from build123d import *

# Parameters (mm, degrees)
SKETCH1_W               = 181
SKETCH1_H               = 90.5
BOSS_EXTRUDE1_DEPTH     = 2.25
SKETCH2_R               = 3.5687
CUT_EXTRUDE1_DEPTH      = 1
CUT_EXTRUDE1_DEPTH_BACK = 91.5


with BuildPart() as part:
    # Sketch1 → Boss-Extrude1 (new body, symmetric)
    with BuildSketch(Plane(origin=(0, 0, 0), x_dir=(0, 0, -1), z_dir=(1, 0, 0))):
        with Locations((0, -45.25)):
            Rectangle(SKETCH1_W, SKETCH1_H)
    extrude(amount=BOSS_EXTRUDE1_DEPTH, both=True)

    # Sketch2 → Cut-Extrude1 (cut, two sides)
    with BuildSketch(Plane(origin=(88.25, 0, 0), x_dir=(0, 0, -1), z_dir=(1, 0, 0))) as cut_extrude1_sk:
        with Locations((0, -69.85)):
            Circle(SKETCH2_R)
        with Locations((69.85, -69.85)):
            Circle(SKETCH2_R)
    extrude(amount=CUT_EXTRUDE1_DEPTH, mode=Mode.SUBTRACT)
    extrude(cut_extrude1_sk.sketch, amount=-CUT_EXTRUDE1_DEPTH_BACK, mode=Mode.SUBTRACT)


solid = part.part
Design review of the part built by this model. Coordinates are the model's own, in mm. Give positions to 0.01 mm unless a question says otherwise; leave off trailing zeros. Loops run counter-clockwise (first coordinate to the right, second up) from the corner with the lowest first, then second, coordinate; pieces in that order, holes last. Notation, with made-up numbers: (80.5, 83) -> (105.5, 83) arc R8 cw to (105.5, 88) -> close; hole circle Ø5 at (43.25, 83.5). An arc over 180 degrees is marked (long way). One line per question, with ' | ' between items. Start each with the question number.
(1) We need section A-A (y = -69.85). State the section outline as (x, z) points, and give its area (3 significant figures).
(2) We need section B-B (z = 0). State the section outline as (x, y) points, and give its area (3 significant figures).
(3) For line 1 (Y direction, x = 0.2, z = -69.85); line 2 (Z direction, x = 0.6, y = -68), list the stretches that pass through material, from the lowest coordinate up.
(4) Insertion check: P1, Ø8, axis at y = -69.85, z = -69.85, coming from the -X side. The pin has a flat end and moves straight along its axis. Give the tip position at first contact, or say it passes through.
(5) Draft analysis for pull direction Y (two halves, no side actions). For faces 1 (the face through (0, -90.5, 1)), 2 (the face through (0.031, -73.016, -71.497)), 3 (the face through (0.031, -73.016, -1.647)), 4 (the face through (0, -46, -90.5)), state which applies: +Y half, -Y half, draft (parallel to the pull), parting line (faces both ways), or undercut.
The answers:
1) outline: (-2.25, -90.5) -> (2.25, -90.5) -> (2.25, -73.42) -> (-2.25, -73.42) -> close; (-2.25, -66.28) -> (2.25, -66.28) -> (2.25, -3.57) -> (-2.25, -3.57) -> close; (-2.25, 3.57) -> (2.25, 3.57) -> (2.25, 90.5) -> (-2.25, 90.5) -> close | area: 750 mm^2
2) outline: (-2.25, -90.5) -> (2.25, -90.5) -> (2.25, -73.42) -> (-2.25, -73.42) -> close; (-2.25, -66.28) -> (2.25, -66.28) -> (2.25, 0) -> (-2.25, 0) -> close | area: 375 mm^2
3) line 1: y = -90.5 to -73.42, -66.28 to 0 | line 2: z = -90.5 to -72.9, -66.8 to -3.05, 3.05 to 90.5
4) P1: stops at x = -2.25
5) face 1: -Y half | face 2: undercut | face 3: undercut | face 4: draft
